Could you check a few things on this model? Use its own coordinates, in mm. Face numbers are marked on the shaded views. Give positions to 0.01 mm unless a question says otherwise; leave off trailing zeros. Loops run counter-clockwise (first coordinate to the right, second up) from the corner with the lowest first, then second, coordinate; pieces in that order, holes last. Notation, with made-up numbers: M 80.25,-17 L 115.25,-17 A26 cw 115.25,9 Z; hole C 6,-15.75 d9. An arc over 180 degrees is marked long. Use CSV: the item, a comma, the result in double quotes.
```python
from build123d import *

# Parameters (mm, degrees)
F0_R     = 21
F0_R_2   = 6
F1_DEPTH = 15
F2_R     = 3


with BuildPart() as f1:
    # F0 (on Top) → F1 (new body)
    with BuildSketch(Plane.XY):
        with BuildLine():
            Line((12.857143, -27.105237), (41.428571, -13.552619))
            ThreePointArc((41.428571, -13.552619), (50, 0), (41.428571, 13.552619))
            Line((41.428571, 13.552619), (12.857143, 27.105237))
            ThreePointArc((12.857143, 27.105237), (0, 30), (-12.857143, 27.105237))
            Line((-12.857143, 27.105237), (-41.428571, 13.552619))
            ThreePointArc((-41.428571, 13.552619), (-50, 0), (-41.428571, -13.552619))
            Line((-41.428571, -13.552619), (-12.857143, -27.105237))
            ThreePointArc((-12.857143, -27.105237), (0, -30), (12.857143, -27.105237))
        make_face()
        Circle(F0_R, mode=Mode.SUBTRACT)
        with Locations((-35, 0)):
            Circle(F0_R_2, mode=Mode.SUBTRACT)
        with Locations((35, 0)):
            Circle(F0_R_2, mode=Mode.SUBTRACT)
    extrude(amount=F1_DEPTH)

    # F2
    f2_edges = [f1.edges().sort_by_distance(p)[0] for p in [
        (-27.142857, -20.328928, 15),
        (-50, 0, 15),
        (-27.142857, 20.328928, 15),
        (0, 30, 15),
        (27.142857, 20.328928, 15),
        (50, 0, 15),
        (27.142857, -20.328928, 15),
        (0, -30, 15),
    ]]
    fillet(f2_edges, radius=F2_R)


solid = f1.part
```
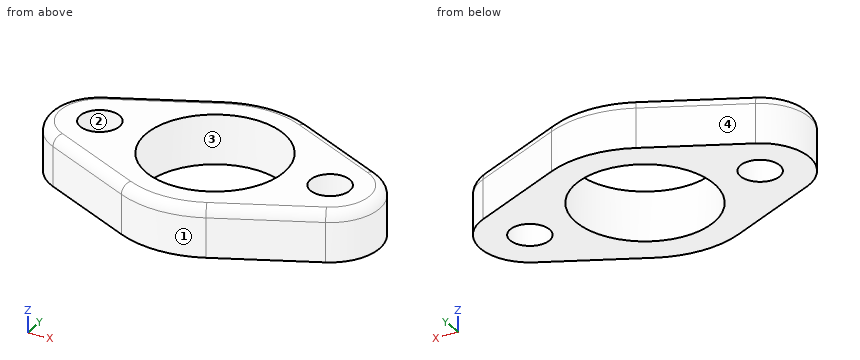
1. I want a section at C-C, the plane z = 10.25. List the corners of the cut face in (x, y) for me, then the cut area to 3 significant figures.
Outcome:
outline,"M -41.43,-13.55 L -12.86,-27.11 A30 ccw 12.86,-27.11 L 41.43,-13.55 A15 ccw 41.43,13.55 L 12.86,27.11 A30 ccw -12.86,27.11 L -41.43,13.55 A15 ccw Z; hole C -35,0 d12; hole C 0,0 d42; hole C 35,0 d12"
area,"2,540 mm2"
2. I want a section at A-A, the plane y = 0. List the corners of the cut face in (x, z) for me, then the cut area to 3 significant figures.
Outcome:
outline,"M -50,0 L -41,0 L -41,15 L -47,15 A3 ccw -50,12 Z; M -29,0 L -21,0 L -21,15 L -29,15 Z; M 21,0 L 29,0 L 29,15 L 21,15 Z; M 41,0 L 50,0 L 50,12 A3 ccw 47,15 L 41,15 Z"
area,"506 mm2"
3. I want a section at B-B, the plane x = 0. List the corners of the cut face in (y, z) for me.
Outcome:
outline,"M -30,0 L -21,0 L -21,15 L -27,15 A3 ccw -30,12 Z; M 21,0 L 30,0 L 30,12 A3 ccw 27,15 L 21,15 Z"
4. If we mould it in two halves opening along X, with no side actions, what happens to the marked faces 1, 2, 3 and 4? For each: +X half, -X half, draft (parallel to the pull), parting line (faces both ways), or undercut.
Outcome:
face 1,"parting line"
face 2,"undercut"
face 3,"undercut"
face 4,"-X half"
5. I'm going to push flat-ended pins straight in: pin 1 Ø8 at (x, z) = (-32.5, 10) entering from +Y; pin 2 Ø4 at (x, z) = (-29, 6) entering from +Y; pin 3 Ø1 at (x, z) = (-39.5, 10.5) entering from -Y. Where does each tip first touch, or does it pass through?
Outcome:
pin 1,"y = 19.69"
pin 2,"y = 20.4"
pin 3,"y = -14.7"
6. Please list where these lines run through material, in increasing order: line 1 (Y direction, x = 0.5, z = 9); line 2 (Y direction, x = -35, z = 8.75); line 3 (X direction, y = -8.5, z = 3.5).
Outcome:
line 1,"-30 to -20.99, 20.99 to 30"
line 2,"-16.6 to -6, 6 to 16.6"
line 3,"-47.36 to -19.2, 19.2 to 47.36"
